The model under review builds one solid part; all positions refer to its coordinate system, in mm. Face numbers are marked on the shaded views. A direction names the side the tool comes from. Coordinates: 2 decimals unless noted, no trailing zeros. Loops run counter-clockwise (first coordinate to the right, second up) from the corner with the lowest first, then second, coordinate; pieces in that order, holes last. Notation, with made-up numbers: (-24.5, 40) - (5.5, 40) arc R18 cw to (5.5, 74) - close; hole circle Ø8 at (-7, 63). An arc over 180 degrees is marked (long way). Answer in a Markdown table with one row per item. Add a question column.
(1) For line 1 along Y through (x, z) = (22.25, -6); line 2 along Y through (x, z) = (23.75, -38); line 3 along Z through (x, y) = (1.75, 13), list the stretches that pass through material, from the lowest coordinate up.
(2) We need section D-D on x = 15.75. Write out the cut boundary in (y, z), plus the area to 3 significant figures.
(3) We need section C-C on y = 12.5. Write out the cut boundary in (x, z).
(4) We need section B-B on y = 7. Write out the cut boundary in (x, z), plus the area to 3 significant figures.
(5) We need section A-A on x = 12.7. Write out the cut boundary in (y, z), plus the area to 3 significant figures.
(6) Machinability: for the marked faces 1, 2 and 3, which of the approach directions +Z, -Z, +X, -X, +Y, -Y give a long, thin tool a straight path to every point of the face, cutting with its end or side? Answer none if there is none.
(7) For P1, Ø6, axis at x = 10.5, z = -8.5, coming from the -Y side; P2, Ø3, axis at y = 13.06, z = -5.99, coming from the +X side; P3, Ø6, axis at x = 19, z = -27.5, coming from the -Y side; P4, Ø3, axis at x = 2, y = 8.5, coming from the -Z side, all flat-tipped, find the tip position at first contact; note any pin that passes through.
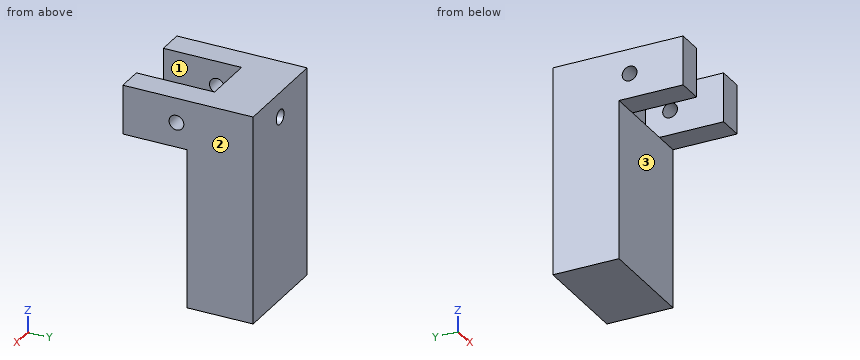
from build123d import *

# Parameters (mm, degrees)
BOSS_EXTRUDE1_DEPTH  = 25.4
SKETCH2_W            = 12.7
SKETCH2_H            = 19.05
CUT_EXTRUDE1_DEPTH   = 11.9888
M3_CLEARANCE_HOLE1_D = 3.6
M3_CLEARANCE_HOLE2_D = 3.6


with BuildPart() as part:
    # Sketch1 → Boss-Extrude1 (new body)
    with BuildSketch(Plane(origin=(0, 0, 0), x_dir=(0, 0, -1), z_dir=(1, 0, 0))):
        Polygon((0, 0), (0, 31.75), (50.8, 31.75), (50.8, 15.6337), (11.9888, 15.6337), (11.9888, 0), align=None)
    extrude(amount=BOSS_EXTRUDE1_DEPTH)

    # Sketch2 → Cut-Extrude1 (cut)
    with BuildSketch(Plane.XY):
        with Locations((12.7, 9.525)):
            Rectangle(SKETCH2_W, SKETCH2_H)
    extrude(amount=-CUT_EXTRUDE1_DEPTH, mode=Mode.SUBTRACT)

    # M3 Clearance Hole1 (through all)
    with Locations(Plane(origin=(25.4, 0, 0), x_dir=(0, 0, -1), z_dir=(1, 0, 0))):
        with Locations((5.9944, 13.0556)):
            Hole(M3_CLEARANCE_HOLE1_D / 2)

    # M3 Clearance Hole2 (through all)
    with Locations(Plane(origin=(0, 31.75, 0), x_dir=(1, 0, 0), z_dir=(0, 1, 0))):
        with Locations((12.7, 5.9944)):
            Hole(M3_CLEARANCE_HOLE2_D / 2)


solid = part.part
Outcome:
| question | item | result |
|---|---|---|
| 1 | line 1 | 0 to 11.26, 14.86 to 31.75 |
| 1 | line 2 | 15.63 to 31.75 |
| 1 | line 3 | -11.99 to -7.79, -4.2 to 0 |
| 2 | outline | (15.63, -50.8) - (31.75, -50.8) - (31.75, 0) - (19.05, 0) - (19.05, -11.99) - (15.63, -11.99) - close |
| 2 | area | 778 mm² |
| 3 | outline | (0, -11.99) - (6.35, -11.99) - (6.35, -7.71) - (0, -7.71) - close; (0, -4.28) - (6.35, -4.28) - (6.35, 0) - (0, 0) - close; (19.05, -11.99) - (25.4, -11.99) - (25.4, -7.71) - (19.05, -7.71) - close; (19.05, -4.28) - (25.4, -4.28) - (25.4, 0) - (19.05, 0) - close |
| 4 | outline | (0, -11.99) - (6.35, -11.99) - (6.35, 0) - (0, 0) - close; (19.05, -11.99) - (25.4, -11.99) - (25.4, 0) - (19.05, 0) - close |
| 4 | area | 152 mm² |
| 5 | outline | (15.63, -50.8) - (31.75, -50.8) - (31.75, -7.79) - (19.05, -7.79) - (19.05, -11.99) - (15.63, -11.99) - close; (19.05, -4.19) - (31.75, -4.19) - (31.75, 0) - (19.05, 0) - close |
| 5 | area | 732 mm² |
| 6 | face 1 | +Z, -Y |
| 6 | face 2 | +Z, -Z, +X, +Y, -Y |
| 6 | face 3 | -Z, +X, -X, -Y |
| 7 | P1 | y = 19.05 |
| 7 | P2 | through |
| 7 | P3 | y = 15.63 |
| 7 | P4 | z = -11.99 |
